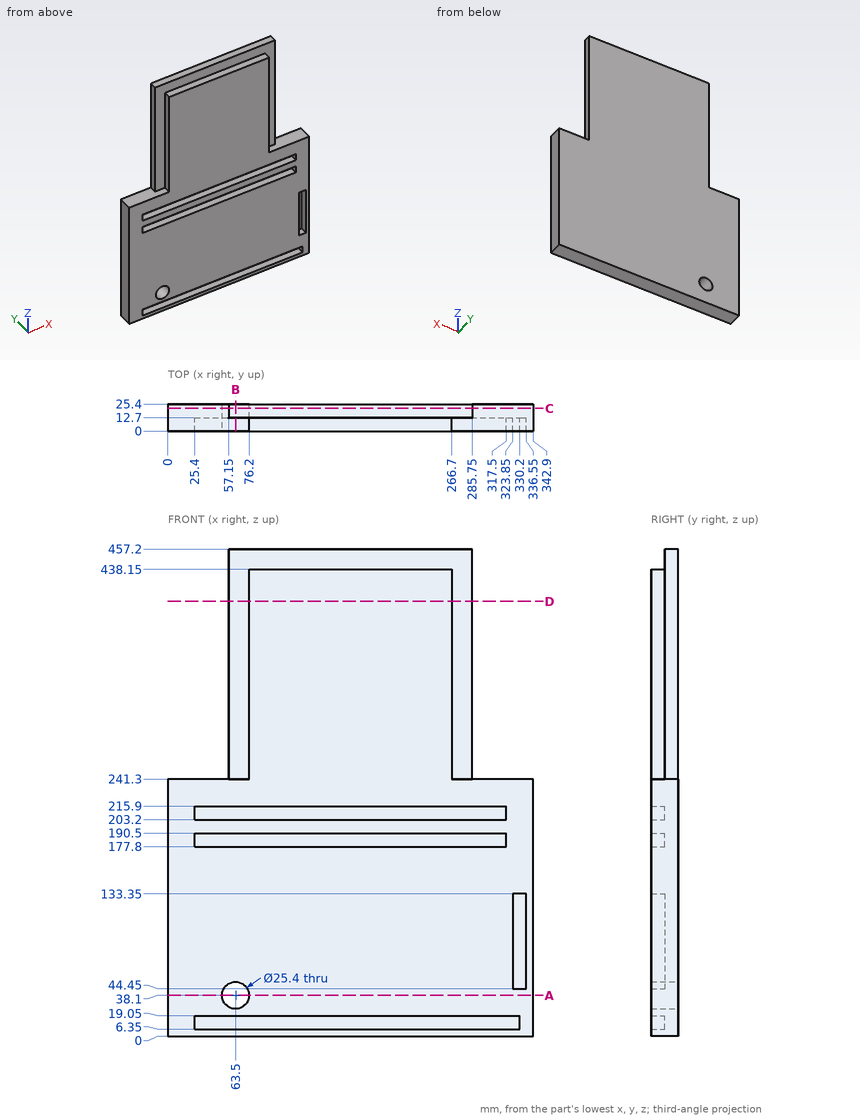
Part print with two shaded views. Sizes in mm from the minimum x, y, z corner. Round coordinates to 2 decimals unless told otherwise and drop trailing zeros. Order: outer loops, then holes, each group sorted by start corner. A loop starts at its lowest first (then second) coordinate and runs counter-clockwise, first axis right, second up. Notation, with made-up numbers: M 66.5,14.25 L 78.5,14.25 A17 cw 78.5,30.25 Z; hole C -40,12 d10. An arc over 180 degrees is marked long. Put each result on its own line as item: value. Start each with the question number.
1. Slice it at A-A on z = 38.1. List the corners of the cut face in (x, y), then the cut area to 3 significant figures.
2. Slice it at C-C on y = 21.25. List the corners of the cut face in (x, z), then the cut area to 3 significant figures.
3. Drop flat-ended pins along their axis: pin 1 (14 mm diameter, centred on x = 240, y = 9.5, fed in from +Z); pin 2 (14 mm diameter, centred on x = 333, y = 4.5, fed in from +Z); pin 3 (10 mm diameter, centred on y = 16.5, z = 378, fed in from -X); pin 4 (6.5 mm diameter, centred on x = 246.5, z = 11, fed in from -Y). Give the stop position or say it passes through.
4. Slice it at B-B on x = 63.5. List the corners of the cut face in (y, z), then the cut area to 3 significant figures.
5. Slice it at D-D on z = 408. List the corners of the cut face in (x, y), then the cut area to 3 significant figures.
6. Drill centre lines: probe 1 along Z at (x, y) = (63.5, 6.5); probe 2 along Z at (x, y) = (120, 9); probe 3 along Z at (x, y) = (63.5, 17.75). Where is each one in solid material? Low to high. Write a range as [from, to].
Findings:
1. outline: M 0,0 L 50.8,0 L 50.8,25.4 L 0,25.4 Z; M 76.2,0 L 342.9,0 L 342.9,25.4 L 76.2,25.4 Z
1. area: 8,060 mm2
2. outline: M 0,0 L 342.9,0 L 342.9,241.3 L 285.75,241.3 L 285.75,457.2 L 57.15,457.2 L 57.15,241.3 L 0,241.3 Z; hole C 63.5,38.1 d25.4
2. area: 132,000 mm2
3. pin 1: z = 457.2
3. pin 2: z = 241.3
3. pin 3: x = 57.15
3. pin 4: y = 12.7
4. outline: M 0,0 L 25.4,0 L 25.4,25.4 L 0,25.4 L 0,19.05 L 12.7,19.05 L 12.7,6.35 L 0,6.35 Z; M 0,50.8 L 25.4,50.8 L 25.4,457.2 L 12.7,457.2 L 12.7,241.3 L 0,241.3 L 0,215.9 L 12.7,215.9 L 12.7,203.2 L 0,203.2 L 0,190.5 L 12.7,190.5 L 12.7,177.8 L 0,177.8 Z
4. area: 7,740 mm2
5. outline: M 57.15,12.7 L 76.2,12.7 L 76.2,0 L 266.7,0 L 266.7,12.7 L 285.75,12.7 L 285.75,25.4 L 57.15,25.4 Z
5. area: 5,320 mm2
6. probe 1: [0, 6.35], [19.05, 25.4], [50.8, 177.8], [190.5, 203.2], [215.9, 241.3]
6. probe 2: [0, 6.35], [19.05, 177.8], [190.5, 203.2], [215.9, 438.15]
6. probe 3: [0, 25.4], [50.8, 457.2]
